Geometry: final body of the model. Coordinates: model frame, mm. Give positions to 0.01 mm unless a question says otherwise; leave off trailing zeros. Order: outer loops, then holes, each group sorted by start corner. A loop starts at its lowest first (then second) coordinate and runs counter-clockwise, first axis right, second up. Notation, with made-up numbers: (18.5, -40) - (34.5, -40) arc R30 ccw to (34.5, -3) - close; hole circle Ø6 at (46.25, 71.25). An arc over 180 degrees is marked (long way). One line per item, written item: value.
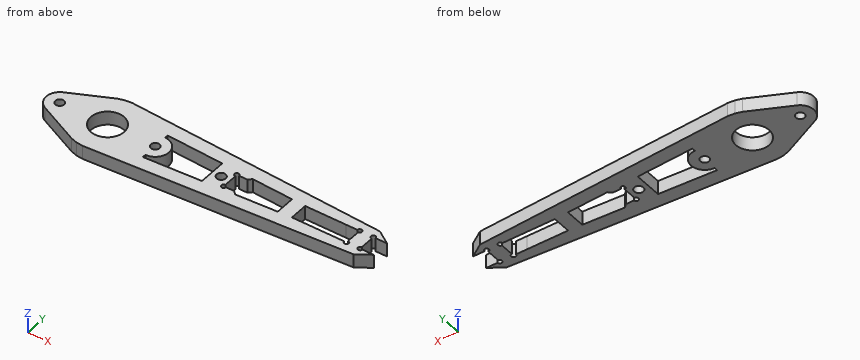
```python
from build123d import *

# Parameters (mm, degrees)
SKETCH_2_R      = 0.999999817
SKETCH_2_R_2    = 0.950000242
SKETCH_2_R_3    = 3.65
EXTRUDE_2_DEPTH = 3


with BuildPart() as part:
    # 草图2 → 凸台-拉伸2 (new body)
    with BuildSketch(Plane.XY):
        with BuildLine():
            Line((57.00000003, 4.00000019), (0, 7.499999832))
            Line((0, 7.499999832), (-1.463177381, 7.355889771))
            Line((-1.463177381, 7.355889771), (-2.870125696, 6.9290963))
            Line((-2.870125696, 6.9290963), (-11.76304094, 2.710484566))
            ThreePointArc((-11.76304094, 2.710484566), (-13.477244136, 0), (-11.76304094, -2.710484566))
            Line((-11.76304094, -2.710484566), (-2.870125696, -6.9290963))
            Line((-2.870125696, -6.9290963), (-1.463177381, -7.355889771))
            Line((-1.463177381, -7.355889771), (0, -7.499999832))
            Line((0, -7.499999832), (57.00000003, -4.00000019))
            Line((57.00000003, -4.00000019), (59.999998659, -2.000000095))
            Line((59.999998659, -2.000000095), (57.500001043, -2.000000095))
            ThreePointArc((57.500001043, -2.000000095), (56.646447675, -2.35355404), (57.00000003, -1.500000013))
            Line((57.00000003, -1.500000013), (57.00000003, 1.500000013))
            ThreePointArc((57.00000003, 1.500000013), (56.646447675, 2.35355404), (57.500001043, 2.000000095))
            Line((57.500001043, 2.000000095), (59.999998659, 2.000000095))
            Line((59.999998659, 2.000000095), (57.00000003, 4.00000019))
        make_face()
        with Locations((25.000000026, 3.041e-06)):
            Circle(SKETCH_2_R, mode=Mode.SUBTRACT)
        with Locations((10.499999852, -1.691e-06)):
            Circle(SKETCH_2_R_2, mode=Mode.SUBTRACT)
        with Locations((-10.499999865, -1.691e-06)):
            Circle(SKETCH_2_R_2, mode=Mode.SUBTRACT)
        Circle(SKETCH_2_R_3, mode=Mode.SUBTRACT)
        with BuildLine():
            Line((41.999999434, 2.002923982), (50.999999046, 2.000000095))
            Line((50.999999046, 2.000000095), (53.500000387, 2.000000095))
            ThreePointArc((53.500000387, 2.000000095), (54.353553756, 2.35355404), (54.000001401, 1.500000013))
            Line((54.000001401, 1.500000013), (54.000001401, -1.500000013))
            ThreePointArc((54.000001401, -1.500000013), (54.353553756, -2.35355404), (53.500000387, -2.000000095))
            Line((53.500000387, -2.000000095), (50.999999046, -2.000000095))
            Line((50.999999046, -2.000000095), (41.999999434, -2.002923982))
            Line((41.999999434, -2.002923982), (41.999999434, 2.002923982))
        make_face(mode=Mode.SUBTRACT)
        with BuildLine():
            Line((27.499999851, 2.000000095), (29.282599688, 2.000000095))
            Line((29.282599688, 2.000000095), (29.999999329, 2.673489275))
            Line((29.999999329, 2.673489275), (39.000000805, 2.170565305))
            Line((39.000000805, 2.170565305), (39.000000805, -2.170565305))
            Line((39.000000805, -2.170565305), (29.999999329, -2.673489275))
            Line((29.999999329, -2.673489275), (29.282599688, -2.000000095))
            Line((29.282599688, -2.000000095), (27.499999851, -2.000000095))
            ThreePointArc((27.499999851, -2.000000095), (26.646446496, -2.353552709), (27.0000007, -1.500000013))
            Line((27.0000007, -1.500000013), (27.0000007, 1.500000013))
            ThreePointArc((27.0000007, 1.500000013), (26.646446496, 2.353552709), (27.499999851, 2.000000095))
        make_face(mode=Mode.SUBTRACT)
        with BuildLine():
            Line((10.499999858, -3.763157874), (10.499999858, -3.000008481))
            ThreePointArc((10.499999858, -3.000008481), (13.500006642, -1.691e-06), (10.499999858, 3.000008481))
            Line((10.499999858, 3.000008481), (10.499999858, 3.763157874))
            Line((10.499999858, 3.763157874), (23.000000045, 3.064652439))
            Line((23.000000045, 3.064652439), (23.000000045, -3.064652439))
            Line((23.000000045, -3.064652439), (10.499999858, -3.763157874))
        make_face(mode=Mode.SUBTRACT)
    extrude(amount=EXTRUDE_2_DEPTH)


solid = part.part
```
1) Section B-B, the plane z = 2.4. Count the separate pieces of the cut face and the enclosed holes in it, then the cut area to 3 significant figures.
Answers below:
separate pieces: 1
enclosed holes: 7
area: 566 mm^2
2) Section A-A, the plane x = 47.5. Return loops of the section in (y, z), then the cut area to 3 significant figures.
Answers below:
outline: (-4.58, 0) - (-2, 0) - (-2, 3) - (-4.58, 3) - close; (2, 0) - (4.58, 0) - (4.58, 3) - (2, 3) - close
area: 15.5 mm^2
3) First-contact query: pin 1 (0.9 mm diameter, centred on x = 47.5, z = 1, fed in from +Y); pin 2 (0.8 mm diameter, centred on y = 3.5, z = 1, fed in from +X); pin 3 (0.9 mm diameter, centred on x = 54, y = -2, fed in from +Z); pin 4 (0.9 mm diameter, centred on y = -0.5, z = 1.5, fed in from +X). Flat tips, straight axial feed; report the tip coordinate or a pass-through.
Answers below:
pin 1: y = 4.61
pin 2: x = 58.35
pin 3: through
pin 4: x = 57
4) Material intervals for line 1 along Y through (x, z) = (0, 2.1); line 2 along Y through (x, z) = (16, 0.35); line 3 along Y through (x, z) = (9.5, 0.85), sorted ascending.
Answers below:
line 1: -7.5 to -3.65, 3.65 to 7.5
line 2: -6.52 to -3.46, 3.46 to 6.52
line 3: -6.92 to 6.92
